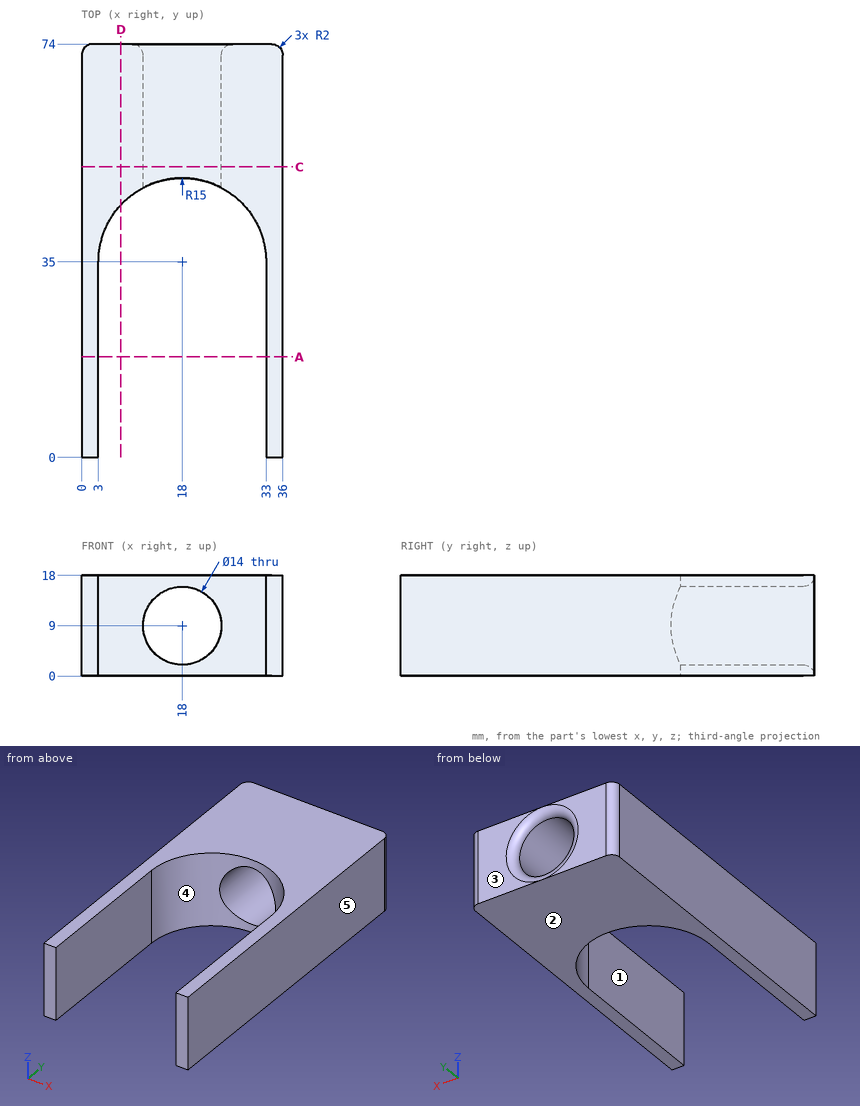
Input: dimensioned drawing with shaded views. Units: mm. Origin: part minimum x, y, z. A direction names the side the tool comes from. Give positions to 0.01 mm unless a question says otherwise; leave off trailing zeros. Loops run counter-clockwise (first coordinate to the right, second up) from the corner with the lowest first, then second, coordinate; pieces in that order, holes last. Notation, with made-up numbers: (48, 85) - (104, 85) arc R24 ccw to (104, 122) - close; hole circle Ø3 at (0.5, -20.75). An arc over 180 degrees is marked (long way). Answer as CSV lines item,"result". Start each with the question number.
(1) Section query C-C (y = 52). Output: boundary loops of the cut face in (x, z).
(2) Pin query (flat end, axial travel): P1, Ø5, axis at x = 27, z = 13.5, coming from the -Y side; P2, Ø8.5, axis at x = 18, z = 9, coming from the +Y side. Return the tip coordinate at first contact, or that it passes through.
(3) Reachability of the marked faces 1 and 2 from +Z, -Z, +X, -X, +Y, -Y: full face, straight path, thin tool, end or side. Return the list, or none.
(4) Mould query, pull axis X, two halves, no side actions, for the marked faces 3, 4 and 5. Classes: +X half, -X half, draft (parallel to the pull), parting line (faces both ways), or undercut.
(5) Section query D-D (x = 7). Output: boundary loops of the cut face in (y, z), and give its area (3 significant figures).
(6) Section query A-A (y = 18). Output: boundary loops of the cut face in (x, z).
(7) Ray query, line 1 along X through (y, z) = (53.25, 9); line 2 along X through (y, z) = (30, 11); line 3 along Z through (x, y) = (18, 61). Return the intervals inside material, ascending. Write a range as [from, to].
Worked answers:
1,outline,"(0, 0) - (36, 0) - (36, 18) - (0, 18) - close; hole circle Ø14 at (18, 9)"
2,P1,"stops at y = 44.63"
2,P2,"passes through"
3,face 1,"+Z, -Z, -Y"
3,face 2,"-Z, +X, -X, +Y, -Y"
4,face 3,"draft"
4,face 4,"undercut"
4,face 5,"+X half"
5,outline,"(45.2, 0) - (74, 0) - (74, 18) - (45.2, 18) - close"
5,area,"518 mm^2"
6,outline,"(0, 0) - (3, 0) - (3, 18) - (0, 18) - close; (33, 0) - (36, 0) - (36, 18) - (33, 18) - close"
7,line 1,"x = [0, 11], [25, 36]"
7,line 2,"x = [0, 3], [33, 36]"
7,line 3,"z = [0, 2], [16, 18]"
